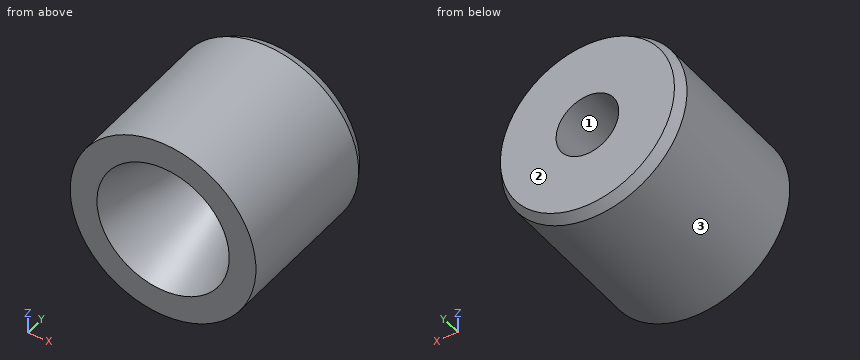
```python
from build123d import *

# Parameters (mm, degrees)
SKETCH1_R           = 8
SKETCH1_R_2         = 2.7
BOSS_EXTRUDE1_DEPTH = 14.05
CHAMFER1_SIZE       = 3
CHAMFER1_SIZE2      = 8.242432258
CHAMFER2_SIZE       = 0.5
CHAMFER2_SIZE2      = 0.866025404


with BuildPart() as part:
    # Sketch1 → Boss-Extrude1 (new body)
    with BuildSketch(Plane(origin=(0, 0, 0), x_dir=(1, 0, 0), z_dir=(0, 1, 0))):
        with Locations(Location((0, 0, 0), (0, 0, 270))):
            Circle(SKETCH1_R)
        with Locations(Location((0, 0, 0), (0, 0, 270))):
            Circle(SKETCH1_R_2, mode=Mode.SUBTRACT)
    extrude(amount=BOSS_EXTRUDE1_DEPTH)

    # Chamfer1
    chamfer1_edges = [part.edges().sort_by_distance(p)[0] for p in [
        (0, 0, -2.7),
    ]]
    chamfer1_side = [part.faces().sort_by_distance(p)[0] for p in [
        (0, 0, -7.77372583),
    ]]
    chamfer(chamfer1_edges, length=CHAMFER1_SIZE, length2=CHAMFER1_SIZE2, reference=chamfer1_side[0])

    # Chamfer2
    chamfer2_edges = [part.edges().sort_by_distance(p)[0] for p in [
        (0, 14.05, -8),
    ]]
    chamfer2_side = [part.faces().sort_by_distance(p)[0] for p in [
        (0, 14.05, -7.77372583),
    ]]
    chamfer(chamfer2_edges, length=CHAMFER2_SIZE, length2=CHAMFER2_SIZE2, reference=chamfer2_side[0])


solid = part.part
```
For this review, take the finished solid that the model builds, in its own axes (mm). Face numbers are marked on the shaded views. Give positions to 0.01 mm unless a question says otherwise; leave off trailing zeros. Write each loop counter-clockwise with the first axis right and the second up, starting at its lowest first coordinate (ties: lowest second). Pieces come first, ordered by that corner, then holes. Notation, with made-up numbers: M 86.5,54.25 L 122.5,54.25 A20 cw 122.5,85.25 Z; hole C -14,12 d3. An arc over 180 degrees is marked long. Answer as a JSON object with one key per item and string values. Group by question number.
Item 1: Consider section A-A on z = 0. Write out the cut boundary in (x, y), plus the area to 3 significant figures.
Item 2: Consider section D-D on y = 3. Write out the cut boundary in (x, z), plus the area to 3 significant figures.
Item 3: Draft analysis for pull direction Z (two halves, no side actions). For the marked faces 1, 2 and 3, state which applies: +Z half, -Z half, draft (parallel to the pull), parting line (faces both ways), or undercut.
Item 4: Consider section B-B on x = 0. Write out the cut boundary in (y, z), plus the area to 3 significant figures.
Item 5: For probe 1 along X at (y, z) = (12.25, 0); probe 2 along Z at (x, y) = (0.25, 6.75); probe 3 along X at (y, z) = (5.5, -2), list the stretches that pass through material, from the lowest coordinate up. Write a range as [from, to].
Item 6: Consider section C-C on y = 6.5. Write out the cut boundary in (x, z), plus the area to 3 significant figures.
Item 7: For pin 1 Ø1 at (y, z) = (9.5, 6) entering from -X; pin 2 Ø4 at (x, y) = (-4, 10) entering from +Z, all flat-tipped, find the tip position at first contact; note any pin that passes through.
Check result:
{
 "1": {"outline": "M -8,0 L -5.7,0 L -2.7,8.24 L -2.7,14.05 L -7.5,14.05 L -8,13.18 Z; M 2.7,8.24 L 5.7,0 L 8,0 L 8,13.18 L 7.5,14.05 L 2.7,14.05 Z", "area": "124 mm^2"},
 "2": {"outline": "C 0,0 d16; hole C 0,0 d9.22", "area": "134 mm^2"},
 "3": {"face 1": "undercut", "face 2": "draft", "face 3": "parting line"},
 "4": {"outline": "M 0,-8 L 13.18,-8 L 14.05,-7.5 L 14.05,-2.7 L 8.24,-2.7 L 0,-5.7 Z; M 0,5.7 L 8.24,2.7 L 14.05,2.7 L 14.05,7.5 L 13.18,8 L 0,8 Z", "area": "124 mm^2"},
 "5": {"probe 1": "x = [-8, -2.7], [2.7, 8]", "probe 2": "z = [-8, -3.23], [3.23, 8]", "probe 3": "x = [-7.75, -3.11], [3.11, 7.75]"},
 "6": {"outline": "C 0,0 d16; hole C 0,0 d6.67", "area": "166 mm^2"},
 "7": {"pin 1": "stops at x = -5.81", "pin 2": "stops at z = 7.75"}
}
